Design review of the part shown in the three views and the two pictorial views. Dimensions are in mm from the part's minimum x, y and z. Round coordinates to 2 decimals unless told otherwise and drop trailing zeros. Write each loop counter-clockwise with the first axis right and the second up, starting at its lowest first coordinate (ties: lowest second). Pieces come first, ordered by that corner, then holes. Notation, with made-up numbers: (20, 66) - (26, 66) arc R10 cw to (26, 74) - close; hole circle Ø3 at (62, 0.25). An arc over 180 degrees is marked (long way). Use one line per item in the form item = value.
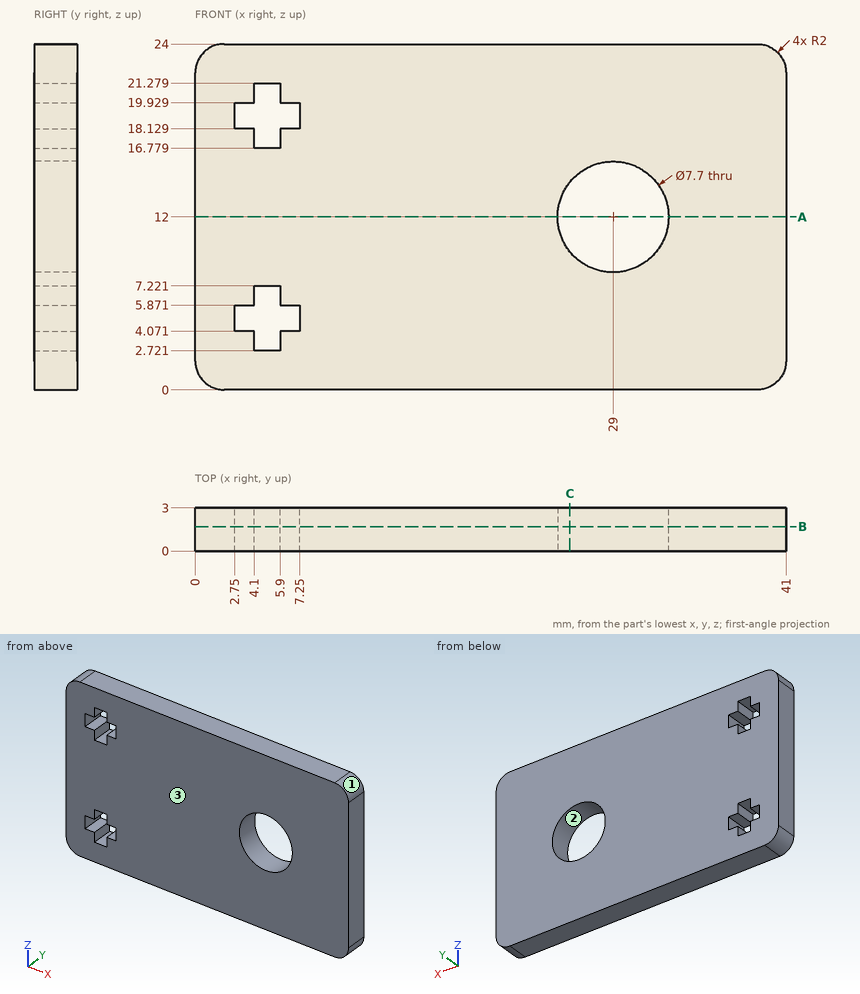
Q1. To check wall thickness, follow line 1 along X through (y, z) = (1.1, 12); line 2 along Z through (x, y) = (6.5, 2.05); line 3 along X through (y, z) = (2.3, 4.25). State the ranges of each line that lie inside material, in increasing order. Write a range as from..to.
Calculated:
line_1 = 0..25.15, 32.85..41
line_2 = 0..4.07, 5.87..18.13, 19.93..24
line_3 = 0..2.75, 7.25..41
Q2. We need section C-C on x = 26. Write out the cut boundary in (y, z).
Calculated:
outline = (0, 0) - (3, 0) - (3, 9.59) - (0, 9.59) - close; (0, 14.41) - (3, 14.41) - (3, 24) - (0, 24) - close
Q3. We need section A-A on z = 12. Write out the cut boundary in (x, y).
Calculated:
outline = (0, 0) - (25.15, 0) - (25.15, 3) - (0, 3) - close; (32.85, 0) - (41, 0) - (41, 3) - (32.85, 3) - close
Q4. We need section B-B on y = 1.7. State how many separate pieces and enclosed holes the cut face has, then the cut area to 3 significant figures.
Calculated:
separate_pieces = 1
enclosed_holes = 3
area = 908 mm2
Q5. Draft analysis for pull direction X (two halves, no side actions). For the marked faces 1, 2 and 3, state which applies: released by +X, released by -X, zero draft, split by the parting line, or undercut.
Calculated:
face_1 = released by +X
face_2 = undercut
face_3 = zero draft
